Design review of the part built by this model. Coordinates are the model's own, in mm. A direction names the side the tool comes from. Give positions to 0.01 mm unless a question says otherwise; leave off trailing zeros. Order: outer loops, then holes, each group sorted by start corner. A loop starts at its lowest first (then second) coordinate and runs counter-clockwise, first axis right, second up.
```python
from build123d import *

# Parameters (mm, degrees)
BOSS_EXTRUDE1_DEPTH = 162.5
SKETCH2_R           = 1.25
CUT_EXTRUDE1_DEPTH  = 8
SKETCH3_R           = 1.25
CUT_EXTRUDE2_DEPTH  = 10


with BuildPart() as part:
    # Sketch1 → Boss-Extrude1 (new body)
    with BuildSketch(Plane.XY):
        Polygon((-7, 9.888282785), (0, 9.888282785), (0, -8.111717215), (-7, -8.111717215), (-7, -6.111717215), (-2, -6.111717215), (-2, 7.888282785), (-7, 7.888282785), align=None)
    extrude(amount=-BOSS_EXTRUDE1_DEPTH)

    # Sketch2 → Cut-Extrude1 (cut, through all)
    with BuildSketch(Plane(origin=(0, 0, 0), x_dir=(0, 0, -1), z_dir=(1, 0, 0))):
        with Locations((5, 3.888282785)):
            Circle(SKETCH2_R)
        with Locations((5, -2.111717215)):
            Circle(SKETCH2_R)
        with Locations((157.5, -2.111717215)):
            Circle(SKETCH2_R)
        with Locations((157.5, 3.888282785)):
            Circle(SKETCH2_R)
    extrude(amount=-CUT_EXTRUDE1_DEPTH, mode=Mode.SUBTRACT)

    # Sketch3 → Cut-Extrude2 (cut)
    with BuildSketch(Plane.XZ.offset(8.111717215)):
        with Locations((-4.5, -37)):
            Circle(SKETCH3_R)
        with Locations((-4.5, -43)):
            Circle(SKETCH3_R)
        with Locations((-4.5, -112)):
            Circle(SKETCH3_R)
        with Locations((-4.5, -118)):
            Circle(SKETCH3_R)
    extrude(amount=-CUT_EXTRUDE2_DEPTH, mode=Mode.SUBTRACT)


solid = part.part
```
1. For line 1 along Y through (x, z) = (-0.6, -157.5); line 2 along Z through (x, y) = (-4.5, -6.75); line 3 along Y through (x, z) = (-2.25, -46.5), list the stretches that pass through material, from the lowest coordinate up.
Recorded:
line 1: y = -8.11 to -3.36, -0.86 to 2.64, 5.14 to 9.89
line 2: z = -162.5 to -119.25, -116.75 to -113.25, -110.75 to -44.25, -41.75 to -38.25, -35.75 to 0
line 3: y = -8.11 to -6.11, 7.89 to 9.89
2. Take a section at B-B (y = 1.25). State the section outline as (x, z) points, then the cut area to 3 significant figures.
Recorded:
outline: (-2, -162.5) - (0, -162.5) - (0, 0) - (-2, 0) - close
area: 325 mm2
3. Draft analysis for pull direction X (two halves, no side actions). For faces 4 (the face through (-5, -6.112, -80)), 5 (the face through (-4.66, -7.13, -41.76)), 6 (the face through (-4.66, -7.13, -110.76)), 7 (the face through (-2, 1, -80)), state which applies: pulls with the +X half, pulls with the -X half, needs draft (parallel to the pull), parting line crosses it, or undercut.
Recorded:
face 4: needs draft
face 5: undercut
face 6: undercut
face 7: pulls with the -X half
4. Machinability: for faces 1 (the face through (-4.66, -7.13, -116.76)), 2 (the face through (-4, 7.888, -80)), 3 (the face through (-3, -8.112, -80)), which of the approach directions +Z, -Z, +X, -X, +Y, -Y give a long, thin tool a straight path to every point of the face, cutting with its end or side? Answer none if there is none.
Recorded:
face 1: -Y
face 2: +Z, -Z, -X
face 3: +Z, -Z, +X, -X, -Y
5. Take a section at A-A (z = -95). State the section outline as (x, y) points.
Recorded:
outline: (-7, -8.11) - (0, -8.11) - (0, 9.89) - (-7, 9.89) - (-7, 7.89) - (-2, 7.89) - (-2, -6.11) - (-7, -6.11) - close
6. For pin 1 (6 mm diameter, centred on y = -2.5, z = -143, fed in from -X); pin 2 (2 mm diameter, centred on x = -4.5, z = -118, fed in from -Y), all flat-tipped, find the tip position at first contact; note any pin that passes through.
Recorded:
pin 1: stops at x = -2
pin 2: stops at y = 7.89
